Here's how the part is built. I have some questions about the finished solid (model axes, mm). Face numbers are marked on the shaded views. A direction names the side the tool comes from. Round coordinates to 2 decimals unless told otherwise and drop trailing zeros. Order: outer loops, then holes, each group sorted by start corner. A loop starts at its lowest first (then second) coordinate and runs counter-clockwise, first axis right, second up. Notation, with made-up numbers: (-28.5, -23) -> (9.5, -23) arc R21 cw to (9.5, -11) -> close; hole circle Ø2 at (25.25, -19.75). An arc over 180 degrees is marked (long way). Use a Markdown table: item, result. Add a question column.
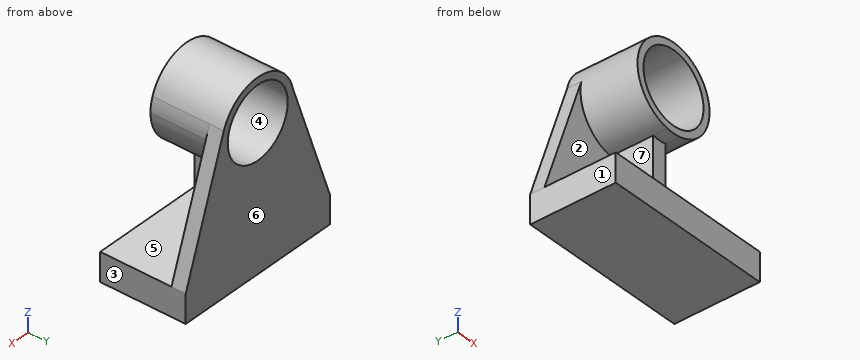
from build123d import *

# Parameters (mm, degrees)
F1_DEPTH = 152.4
F2_DEPTH = 25.4
F4_DEPTH = 101.6
F5_W     = 25.4
F5_H     = 129.54
F6_DEPTH = 101.6
F7_R     = 63.5
F8_DEPTH = 127.001


with BuildPart() as f1:
    # F0 (on Front) → F1 (new body)
    with BuildSketch(Plane.XZ):
        Polygon((-152.4, 0), (-152.4, -50.8), (152.4, -50.8), (152.4, 0), (12.7, 0), (-12.7, 0), align=None)
    extrude(amount=F1_DEPTH)

    # F0 (on Front) → F2 (join)
    with BuildSketch(Plane.XZ):
        Polygon((-152.4, 0), (-152.4, -50.8), (152.4, -50.8), (152.4, 0), (12.7, 0), (-12.7, 0), align=None)
        with BuildLine():
            Line((-74.3468107782, 219.9030454442), (-152.4, 0))
            Line((-152.4, 0), (-12.7, 0))
            Line((-12.7, 0), (-12.7, 128.0657867546))
            ThreePointArc((-12.7, 128.0657867546), (-63.2677432628, 160.7308033696), (-74.3468107782, 219.9030454442))
        make_face()
        with BuildLine():
            Line((12.7, 0), (152.4, 0))
            Line((152.4, 0), (71.8681340167, 228.5260994423))
            ThreePointArc((71.8681340167, 228.5260994423), (75.109226504, 216.0469488193), (76.2, 203.2))
            ThreePointArc((76.2, 203.2), (58.1987113259, 154.0131115032), (12.7, 128.0657867546))
            Line((12.7, 128.0657867546), (12.7, 0))
        make_face()
        with BuildLine():
            Line((-68.2402594432, 237.1073294603), (-74.3468107782, 219.9030454442))
            ThreePointArc((-74.3468107782, 219.9030454442), (-63.2677432628, 160.7308033696), (-12.7, 128.0657867546))
            ThreePointArc((-12.7, 128.0657867546), (0, 127), (12.7, 128.0657867546))
            ThreePointArc((12.7, 128.0657867546), (58.1987113259, 154.0131115032), (76.2, 203.2))
            ThreePointArc((76.2, 203.2), (75.109226504, 216.0469488193), (71.8681340167, 228.5260994423))
            ThreePointArc((71.8681340167, 228.5260994423), (4.6582985773, 279.257479937), (-68.2402594432, 237.1073294603))
        make_face()
        with BuildLine():
            ThreePointArc((-68.2402594432, 237.1073294603), (-71.810618962, 228.6887230809), (-74.3468107782, 219.9030454442))
            Line((-74.3468107782, 219.9030454442), (-68.2402594432, 237.1073294603))
        make_face()
    extrude(amount=F2_DEPTH)

    # F3 (on face) → F4 (join)
    with BuildSketch(Plane.XZ.offset(25.4)):
        with BuildLine():
            ThreePointArc((12.7, 128.0657867546), (58.1987113259, 154.0131115032), (76.2, 203.2))
            ThreePointArc((76.2, 203.2), (75.109226504, 216.0469488193), (71.8681340167, 228.5260994423))
            ThreePointArc((71.8681340167, 228.5260994423), (-4.4861146536, 279.2678300947), (-74.3468107782, 219.9030454442))
            ThreePointArc((-74.3468107782, 219.9030454442), (-63.2677432628, 160.7308033696), (-12.7, 128.0657867546))
            ThreePointArc((-12.7, 128.0657867546), (0, 127), (12.7, 128.0657867546))
        make_face()
    extrude(amount=F4_DEPTH)

    # F5 (on Front) → F6 (join)
    with BuildSketch(Plane.XZ):
        with Locations((0, 64.77)):
            Rectangle(F5_W, F5_H)
    extrude(amount=F6_DEPTH)

    # F7 (on face) → F8 (cut, through all)
    with BuildSketch(Plane.XZ.offset(127)):
        with Locations((0, 203.2)):
            Circle(F7_R)
    extrude(amount=-F8_DEPTH, mode=Mode.SUBTRACT)


solid = f1.part
(1) I want a section at B-B on x = 0. List the corners of the cut face in (y, z) for me, and give its area (3 significant figures).
(2) I want a section at D-D on z = 257. List the corners of the cut face in (x, y) for me, and give its area (3 significant figures).
(3) Please list where these lines run through material, in increasing order: probe 1 along Z at (x, y) = (0, -89.5); probe 2 along Z at (x, y) = (-25.5, -38.5); probe 3 along Z at (x, y) = (16, -100). Write a range as from..to.
(4) On a 3-axis mill with a long thin cutter (end or side, diameter ignored), from which of +Z, -Z, +X, -X, +Y, -Y can I reach the whole of each face in a straight line? I mean the marked faces 5, 6 and 7. Say none if no direction works.
(5) I want a section at A-A on y = -114.5. List the corners of the cut face in (x, z) for me.
(6) I'm going to push flat-ended pins straight in: P1, Ø8, axis at x = 73.5, y = -126.5, coming from the +Z side; P2, Ø7.5, axis at x = -5, z = 66.5, coming from the -Y side; P3, Ø1, axis at y = -44, z = 209, coming from the +X side. Where does each tip first touch, or does it pass through?
(7) I want a section at C-C on y = -15. List the corners of the cut face in (x, z) for me, and give its area (3 significant figures).
(8) If we mould it in two halves opening along X, with no side actions, what happens to the marked faces 1, 2, 3 and 4? For each: pulls with the +X half, pulls with the -X half, needs draft (parallel to the pull), parting line crosses it, or undercut.
Output:
| question | item | result |
|---|---|---|
| 1 | outline | (-152.4, -50.8) -> (0, -50.8) -> (0, 139.7) -> (-127, 139.7) -> (-127, 127) -> (-101.6, 127) -> (-101.6, 0) -> (-152.4, 0) -> close; (-127, 266.7) -> (0, 266.7) -> (0, 279.4) -> (-127, 279.4) -> close |
| 1 | area | 23,900 mm² |
| 2 | outline | (-53.96, -127) -> (-33.73, -127) -> (-33.73, 0) -> (-53.96, 0) -> close; (33.73, -127) -> (53.96, -127) -> (53.96, 0) -> (33.73, 0) -> close |
| 2 | area | 5,140 mm² |
| 3 | probe 1 | -50.8..139.7, 266.7..279.4 |
| 3 | probe 2 | -50.8..0, 131.39..145.05, 261.35..275.01 |
| 3 | probe 3 | -50.8..0, 128.7..141.75, 264.65..277.7 |
| 4 | face 5 | -Y |
| 4 | face 6 | +Z, -Z, +X, -X, +Y |
| 4 | face 7 | -X, -Y |
| 5 | outline | (-152.4, -50.8) -> (152.4, -50.8) -> (152.4, 0) -> (-152.4, 0) -> close; circle Ø152.4 at (0, 203.2); hole circle Ø127 at (0, 203.2) |
| 6 | P1 | z = 234.44 |
| 6 | P2 | y = -101.6 |
| 6 | P3 | x = 76.02 |
| 7 | outline | (-152.4, -50.8) -> (152.4, -50.8) -> (152.4, 0) -> (71.87, 228.53) arc R76.2 ccw to (-74.35, 219.9) -> (-152.4, 0) -> close; hole circle Ø127 at (0, 203.2) |
| 7 | area | 59,300 mm² |
| 8 | face 1 | pulls with the -X half |
| 8 | face 2 | needs draft |
| 8 | face 3 | pulls with the +X half |
| 8 | face 4 | undercut |
